Here's how the part is built. I have some questions about the finished solid (model axes, mm). Face numbers are marked on the shaded views. Coordinates: 2 decimals unless noted, no trailing zeros. Write each loop counter-clockwise with the first axis right and the second up, starting at its lowest first coordinate (ties: lowest second). Pieces come first, ordered by that corner, then holes.
Item 1: If I drill on line 1 (X direction, y = 15.25, z = -20); line 2 (X direction, y = 8.75, z = -17.5); line 3 (Z direction, x = -21.5, y = 11.25), over which ranges is the centre line in solid material (lowest first)?
Item 2: If we section it at C-C (x = 9): Please give me the cut outline in (y, z), then the cut area to 3 significant figures.
Item 3: We'd pull the mould along X, two halves only. Please class the marked faces 1, 2, 3 and 4: +X half, -X half, draft (parallel to the pull), parting line (faces both ways), or undercut.
Item 4: I'm going to push flat-ended pins straight in: pin 1 Ø1.2 at (x, y) = (0, 4.5) entering from +Z; pin 2 Ø3 at (y, z) = (4.5, -24.5) entering from +X; pin 3 Ø5 at (x, z) = (2, -49) entering from +Y. Where does each tip first touch, or does it pass through?
Item 5: If we section it at A-A (y = 10): Count the separate pieces of the cut face and the enclosed holes in it, then the cut area to 3 significant figures.
Item 6: If we section it at B-B (z = -9): Please give me the cut outline in (x, y).
Autodesk Inventor part; units mm, degrees
ref_plane "YZ Plane" through (0, 0, 0) normal (1, 0, 0) x (0, 1, 0)
ref_plane "XZ Plane" through (0, 0, 0) normal (0, 1, 0) x (-1, 0, 0)
ref_plane "XY Plane" through (0, 0, 0) normal (0, 0, 1) x (1, 0, 0)
sketch "Boceto1" plane through (0, 0, 0) normal (0, 1, 0) x (-1, 0, 0)
  line L0 (26, -66) -> (49, -66)
  line L1 (0, -87) -> (0, 0) construction
  line L2 (49, 0) -> (49, -87)
  line L3 (-49, 0) -> (49, 0)
  line L4 (-49, -87) -> (-49, 0)
  line L5 (49, -87) -> (-49, -87)
  line L6 (26, -87) -> (26, -66)
  circle A0 centre (-41.5, -7.5) radius 1.75
  line L7 (49, -12) -> (-49, -12) construction
  circle A1 centre (41.5, -7.5) radius 1.75
  line L8 (-26, -66) -> (-49, -66)
  line L9 (-26, -87) -> (-26, -66)
  line L10 (44.5, -24.05) -> (28.5, -24.05)
  line L11 (28.5, -24.05) -> (28.5, -13.05)
  line L12 (28.5, -13.05) -> (44.5, -13.05)
  line L13 (44.5, -13.05) -> (44.5, -24.05)
  line L14 (42.5, -23.55) -> (31.5, -23.55)
  line L15 (31.5, -14.85) -> (42.5, -14.85)
  line L16 (42.5, -14.85) -> (42.5, -23.55)
  circle A2 centre (30.2, -19.25) radius 1.05
  line L17 (31.5, -14.85) -> (31.5, -23.55)
  line L18 (-42.5, -23.55) -> (-31.5, -23.55)
  line L19 (-42.5, -14.85) -> (-42.5, -23.55)
  line L20 (-31.5, -14.85) -> (-42.5, -14.85)
  line L21 (-31.5, -14.85) -> (-31.5, -23.55)
  circle A3 centre (-30.2, -19.25) radius 1.05
  circle A4 centre (13, -21.5) radius 2.5
  circle A5 centre (-13, -21.5) radius 2.5
  circle A6 centre (16, -70) radius 2.5
  circle A7 centre (-16, -70) radius 2.5
  dimension "d0" = 3.5
  dimension "d1" = 0
  dimension "d2" = 87
  dimension "d3" = 21
  dimension "d4" = 12
  dimension "d5" = 23
  dimension "d6" = 98
  dimension "d7" = 7.5
  dimension "d8" = 7.5
  dimension "d9" = 79.5
  dimension "d10" = 2.1
  dimension "d11" = 9
  dimension "d12" = 11
  dimension "d13" = 16
  dimension "d14" = 1
  dimension "d15" = 3.6
  dimension "d16" = 2.1
  dimension "d17" = 1.3
  dimension "d18" = 5
  dimension "d19" = 36
  dimension "d20" = 9.5
  dimension "d21" = 5
  dimension "d22" = 17
  dimension "d23" = 10
  dimension "d24" = 8.7
  dimension "d25" = 4.3
  dimension "d26" = 4
  dimension "d27" = 11
  dimension "d28" = 54
  dimension "d29" = 2.85
extrude "Base" add sketch "Boceto1" along normal blind 1.5 contours L6 L5 L9 L8 L4 L3 L2 L0 | L10 L11 L12 L13
sketch "Boceto2" plane through (-49, 0, -66) normal (-1, 0, 0) x (0, 0, 1)
  line L0 (66, 0) -> (0, 0)
  line L1 (66, 0) -> (65.1357, 1.5)
  line L2 (66, 0) -> (67.7312, 0) construction
  line L3 (65.1357, 1.5) -> (66, 1.5)
  line L4 (66, 0) -> (66, 1.5)
  line L5 (66, 1.5) -> (66, 0)
  dimension "d32" = 119.95
extrude "Angulo Base" cut sketch "Boceto2" against normal blind 98
sketch "Boceto3" plane through (-49, 0, -66) normal (-1, 0, 0) x (0, 0, 1)
  line L0 (0, 0) -> (66, 0)
  line L1 (51.8028, 0) -> (66, 0)
  line L2 (66, 0) -> (51.8028, 24.6399)
  line L3 (51.8028, 24.6399) -> (51.8028, 0)
  line L4 (66, 0) -> (65.1357, 1.5)
  dimension "d35" = 0
extrude "Extrusión3" add sketch "Boceto3" against normal blind 98
sketch "Boceto4" plane through (-49, 1.5, -14.1972) normal (0, 0, -1) x (-1, 0, 0)
  line L0 (-55.5, 19.6399) -> (-42.5, 19.6399)
  line L1 (-42.5, 19.6399) -> (-42.5, 0.9399)
  line L2 (-42.5, 0.9399) -> (-55.5, 0.9399)
  line L3 (-55.5, 0.9399) -> (-55.5, 19.6399)
  line L4 (-54.6, 10.4399) -> (-43.4, 10.4399)
  line L5 (-43.4, 10.4399) -> (-43.4, 4.8399)
  line L6 (-43.4, 4.8399) -> (-54.6, 4.8399)
  line L7 (-54.6, 4.8399) -> (-54.6, 10.4399)
  line L8 (0, 23.1399) -> (0, 0)
  line L9 (-98, 0) -> (-98, 23.1399)
  line L10 (0, 23.1399) -> (-98, 23.1399)
  line L11 (0, 0) -> (-98, 0)
  point P0 (-49, -1.5)
  dimension "d38" = 13
  dimension "d39" = 0.9
  dimension "d40" = 0.9
  dimension "d41" = 3.9
  dimension "d42" = 5.6
  dimension "d43" = 18.7
  dimension "d44" = 42.5
  dimension "d45" = 42.5
  dimension "d46" = 3.5
  dimension "d93" = 0.9399
extrude "Extrusión4" cut sketch "Boceto4" against normal mid plane 76.25 contours L4 L5 L6 L7
sketch "Boceto5" plane through (-49, 1.5, -14.1972) normal (0, 0, -1) x (-1, 0, 0)
  line L0 (-54.6, 19.64) -> (-43.4, 19.64)
  line L1 (-43.4, 19.64) -> (-43.4, 4.84)
  line L2 (-43.4, 4.84) -> (-54.6, 4.84)
  line L3 (-54.6, 4.84) -> (-54.6, 19.64)
  line L4 (-54.6, 4.8399) -> (-54.6, 10.4399)
  line L5 (-43.4, 10.4399) -> (-43.4, 4.8399)
  line L6 (-43.4, 4.8399) -> (-54.6, 4.8399)
  line L7 (-75, 0) -> (-23, 0)
  line L8 (0, 23.1399) -> (-98, 23.1399)
  point P0 (-49, -1.5)
  dimension "d49" = 11.2
  dimension "d50" = 14.8
  dimension "d76" = 4.84
extrude "Extrusión5" cut sketch "Boceto5" against normal mid plane 1.5
sketch "Boceto6" plane through (0, 1.5, 0) normal (0, 1, 0) x (1, 0, 0)
  line L0 (6.5, 13.7984) -> (-6.5, 13.7984)
  line L1 (-6.5, 13.7984) -> (-6.5, 13.8318)
  line L2 (-6.5, 13.8318) -> (6.5, 13.8318)
  line L3 (6.5, 13.8318) -> (6.5, 13.7984)
  line L4 (-6.5, 13.8318) -> (6.5, 13.8318)
  line L5 (6.5, 13.8318) -> (6.5, 18.6972)
  line L6 (6.5, 18.6972) -> (-6.5, 18.6972)
  line L7 (-6.5, 18.6972) -> (-6.5, 13.8318)
  line L8 (-49, 14.1972) -> (49, 14.1972)
  point P0 (0, 0)
  point P1 (-6.5, 14.1972)
  point P2 (6.5, 14.1972)
  dimension "d53" = 13
  dimension "d54" = 4.5
extrude "Extrusión6" add sketch "Boceto6" along normal blind 20 contours L8 L7 L6 L5
sketch "Boceto7" plane through (6.5, 1.5, -18.6972) normal (0, 0, -1) x (-1, 0, 0)
  line L0 (0.9, 10.916) -> (12.1, 10.916)
  line L1 (12.1, 10.916) -> (12.1, 4.84)
  line L2 (12.1, 4.84) -> (0.9, 4.84)
  line L3 (0.9, 4.84) -> (0.9, 10.916)
  line L4 (13, 0) -> (0, 0)
  line L5 (0, 0) -> (0, 20)
  line L6 (0.9, 20) -> (12.1, 20)
  line L7 (12.1, 20) -> (12.1, 15.894)
  line L8 (12.1, 15.894) -> (0.9, 15.894)
  line L9 (0.9, 15.894) -> (0.9, 20)
  line L10 (0, 20) -> (13, 20)
  point P0 (6.5, -1.5)
  dimension "d57" = 4.84
  dimension "d58" = 6.076
  dimension "d59" = 11.2
  dimension "d60" = 0.9
  dimension "d61" = 4.978
  dimension "d62" = 11.2
  dimension "d63" = 0.9
  dimension "d64" = 0
extrude "Extrusión7" cut sketch "Boceto7" against normal blind 5.25
sketch "Boceto8" plane through (-5.6, 17.394, -18.6972) normal (0, 1, 0) x (1, 0, 0)
  line L0 (0, 0) -> (0, -4.5)
  line L1 (0, -4.5) -> (11.2, -4.5)
  line L2 (11.2, -4.5) -> (11.2, -0.7)
  line L3 (11.2, -0.7) -> (0, -0.7)
  line L4 (0, -0.7) -> (0, -4.5)
  point P0 (5.6, -18.6972)
  point P1 (0, -0.7)
  dimension "d67" = 3.8
  dimension "d68" = 11.2
extrude "Extrusión8" cut sketch "Boceto8" against normal blind 10.054
sketch "Boceto9" plane through (-5.6, 6.34, -18.6972) normal (0, 1, 0) x (1, 0, 0)
  line L0 (11.2, 0) -> (11.2, -0.7)
  line L1 (0, 0) -> (0, -4.5)
  line L2 (11.2, -0.7) -> (0, -0.7)
  line L3 (0, -0.7) -> (0, -1.7)
  line L4 (0, -1.7) -> (11.2, -1.7)
  line L5 (11.2, -1.7) -> (11.2, -0.7)
  point P0 (5.6, -18.6972)
  dimension "d77" = 1
extrude "Extrusión9" cut sketch "Boceto9" against normal blind 3.9
sketch "Boceto14" plane through (0, 1.5, 0) normal (0, 1, 0) x (1, 0, 0)
  line L0 (6.5, 14.1972) -> (6.5, 18.6972)
  line L1 (-6.5, 14.1972) -> (6.5, 14.1972)
  line L2 (6.5, 14.1972) -> (6.5, 18.6972)
  line L3 (6.5, 18.6972) -> (-6.5, 18.6972)
  line L4 (-6.5, 18.6972) -> (-6.5, 14.1972)
  line L5 (39.9859, 2.7887) -> (25.4113, 2.7887)
  line L6 (25.4113, 2.7887) -> (18.1896, 18.2757)
  line L7 (39.9859, 2.7887) -> (32.7642, 18.2757)
  line L8 (34.666, 14.1972) -> (39.9859, 2.7887)
  line L9 (18.1896, 18.2757) -> (30.1611, 23.8581)
  line L10 (18.1896, 18.2757) -> (35.316, 18.2757) construction
  line L11 (32.7642, 18.2757) -> (30.1611, 23.8581)
  line L12 (25.4113, 2.7887) -> (37.326, 8.493)
  line L13 (-5.6, 17.9972) -> (5.6, 17.9972)
  line L14 (5.6, 18.6972) -> (5.6, 14.1972)
  line L15 (20.0915, 14.1972) -> (34.666, 14.1972)
  line L16 (29.6412, 22.8433) -> (33.673, 14.1972)
  line L17 (19.3012, 18.0217) -> (29.6412, 22.8433)
  line L18 (19.3012, 18.0217) -> (21.0845, 14.1972)
  line L19 (20.0915, 14.1972) -> (21.0845, 14.1972)
  line L20 (33.673, 14.1972) -> (34.666, 14.1972)
  line L21 (0, 0) -> (0, 87)
  line L22 (26, 87) -> (-26, 87)
  line L23 (-25.4113, 2.7887) -> (-18.1896, 18.2757)
  line L24 (-39.9859, 2.7887) -> (-32.7642, 18.2757)
  line L25 (-18.1896, 18.2757) -> (-30.1611, 23.8581)
  line L26 (-18.1896, 18.2757) -> (-35.316, 18.2757) construction
  line L27 (-32.7642, 18.2757) -> (-30.1611, 23.8581)
  line L28 (-25.4113, 2.7887) -> (-37.326, 8.493)
  line L29 (-20.0915, 14.1972) -> (-34.666, 14.1972)
  line L30 (-29.6412, 22.8433) -> (-33.673, 14.1972)
  line L31 (-19.3012, 18.0217) -> (-29.6412, 22.8433)
  line L32 (-19.3012, 18.0217) -> (-21.0845, 14.1972)
  line L33 (-20.0915, 14.1972) -> (-21.0845, 14.1972)
  dimension "d94" = 13
  dimension "d95" = 4.5
  dimension "d96" = 17.088
  dimension "d97" = 17.088
  dimension "d98" = 25
  dimension "d99" = 0.7
  dimension "d100" = 0.9
  dimension "d101" = 90
  dimension "d103" = 0.9
  dimension "d104" = 0.7
extrude "Extrusión11" add sketch "Boceto14" along normal up to surface (20 mm away) contours L6 L9 L11 L7 L15 L16 L17 L18 | L29 L32 L31 L30 L24 L27 L25 L23
sketch "Boceto15" plane through (30.1611, 1.5, -23.8581) normal (-0.4226, 0, -0.9063) x (-0.9063, 0, 0.4226)
  point P0 (37.4181, -1.5)
equation "\"Radio_pliegue\" = Grosor"
equation "\"Anchura_desahogo_plegado\" = Grosor"
equation "\"Profundidad_desahogo_plegado\" = 0.5 * Grosor"
equation "\"Tamaño_destalonado\" = 4 * Grosor"
equation "\"Remanente_mínimo\" = 2 * Grosor"
equation "\"Radiodetransición\" = Radio_pliegue"
equation "\"Tamaño_de_radio_de_Jacobi\" = Radio_pliegue"
equation "\"TamañoSeparación\" = Grosor"
properties part number "Onixium3"
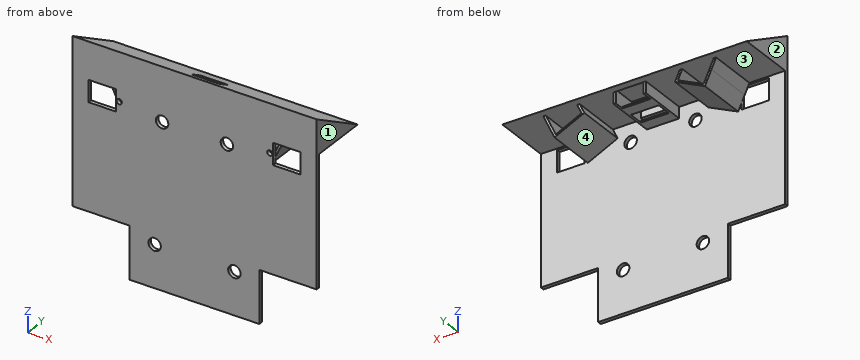
Answer list:
1. line 1: x = -31.96 to -30.97, -23.54 to -21.89, 21.89 to 23.54, 30.97 to 31.96
1. line 2: x = -33.13 to -32.13, -19.54 to -18.55, -6.5 to -5.6, 5.6 to 6.5, 18.55 to 19.54, 32.13 to 33.13
1. line 3: z = -19.82 to -19.05, -14.2 to -6.48
2. outline: (0, -87) - (1.5, -87) - (1.5, -14.2) - (24.64, -14.2) - (1.5, -0.86) - (0, 0) - close
2. area: 284 mm2
3. face 1: +X half
3. face 2: -X half
3. face 3: undercut
3. face 4: undercut
4. pin 1: stops at z = -2.25
4. pin 2: stops at x = 30.56
4. pin 3: stops at y = 1.5
5. separate pieces: 2
5. enclosed holes: 2
5. area: 784 mm2
6. outline: (-49, 0) - (49, 0) - (49, 15.62) - (-49, 15.62) - close; hole (-5.6, 6.34) - (5.6, 6.34) - (5.6, 11.94) - (-5.6, 11.94) - close
